Here's the drawing with two shaded views (mm, measured from the low corner). I have some questions. A direction names the side the tool comes from. Give positions to 0.01 mm unless a question says otherwise; leave off trailing zeros. Write each loop counter-clockwise with the first axis right and the second up, starting at its lowest first coordinate (ties: lowest second). Pieces come first, ordered by that corner, then holes.
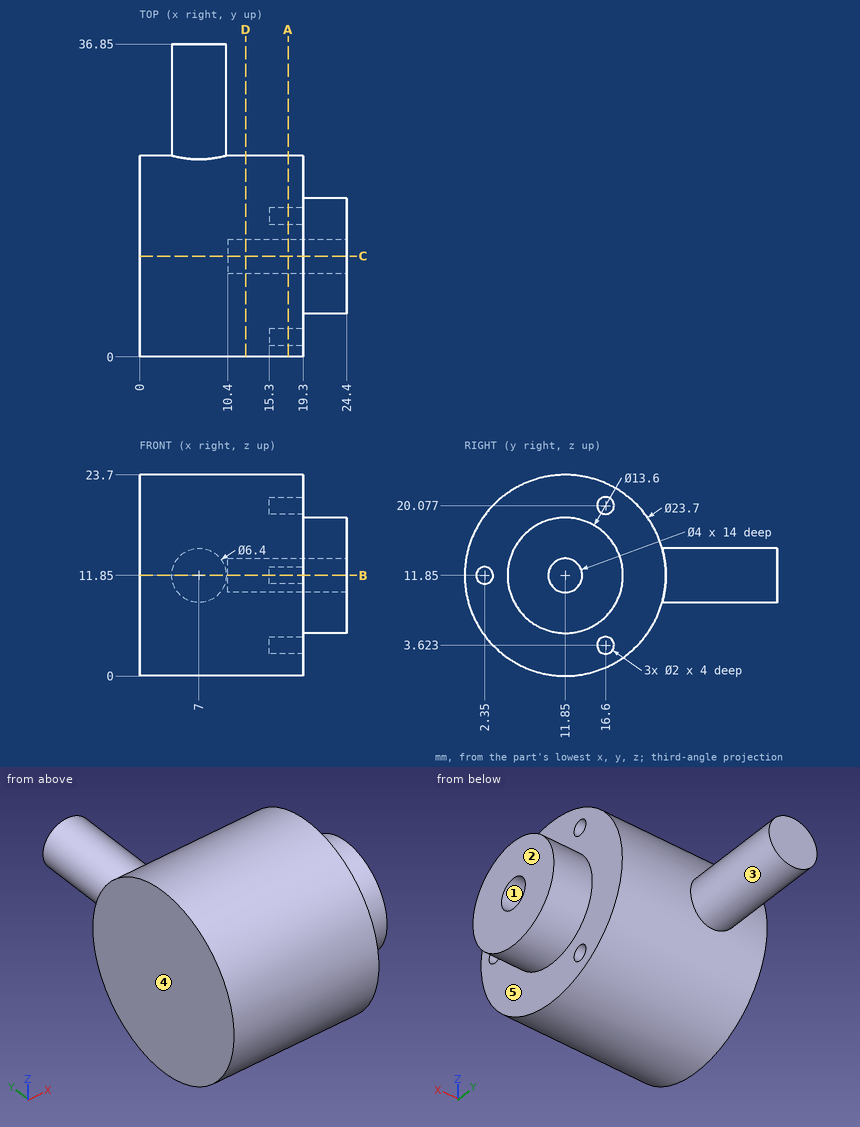
(1) Imagine slicing it at B-B, the plane z = 11.85. Write out the boundary of the cut face in (x, y), plus the area to 3 significant figures.
Returned:
outline: (0, 0) - (19.3, 0) - (19.3, 1.35) - (15.3, 1.35) - (15.3, 3.35) - (19.3, 3.35) - (19.3, 5.05) - (24.4, 5.05) - (24.4, 9.85) - (10.4, 9.85) - (10.4, 13.85) - (24.4, 13.85) - (24.4, 18.65) - (19.3, 18.65) - (19.3, 23.7) - (10.2, 23.7) - (10.2, 36.85) - (3.8, 36.85) - (3.8, 23.7) - (0, 23.7) - close
area: 547 mm2
(2) Imagine slicing it at C-C, the plane y = 11.85. Write out the boundary of the cut face in (x, z), plus the area to 3 significant figures.
Returned:
outline: (0, 0) - (19.3, 0) - (19.3, 5.05) - (24.4, 5.05) - (24.4, 9.85) - (10.4, 9.85) - (10.4, 13.85) - (24.4, 13.85) - (24.4, 18.65) - (19.3, 18.65) - (19.3, 23.7) - (0, 23.7) - close
area: 471 mm2
(3) If we mould it in two halves opening along Z, with no side actions, what happens to the marked faces 1, 2 and 3? For each: +Z half, -Z half, draft (parallel to the pull), parting line (faces both ways), or undercut.
Returned:
face 1: undercut
face 2: draft
face 3: parting line
(4) Will these pins go through, and if not, where does the flat tip stop? P1, Ø2.5, axis at y = 16.6, z = 20.08, coming from the +X side; P2, Ø1.5, axis at x = 12.5, z = 3.5, coming from the +Y side; P3, Ø1.6, axis at y = 16.6, z = 3.62, coming from the +X side; P4, Ø8, axis at x = 10, z = 15.5, coming from the -Y side.
Returned:
P1: stops at x = 19.3
P2: stops at y = 20.94
P3: stops at x = 15.3
P4: stops at y = 0
(5) Imagine slicing it at D-D, the plane x = 12.5. Write out the boundary of the cut face in (y, z), plus the area to 3 significant figures.
Returned:
outline: circle Ø23.7 at (11.85, 11.85); hole circle Ø4 at (11.85, 11.85)
area: 429 mm2
(6) Imagine slicing it at A-A, the plane x = 17.5. Write out the boundary of the cut face in (y, z), plus the area to 3 significant figures.
Returned:
outline: circle Ø23.7 at (11.85, 11.85); hole circle Ø2 at (2.35, 11.85); hole circle Ø4 at (11.85, 11.85); hole circle Ø2 at (16.6, 3.62); hole circle Ø2 at (16.6, 20.08)
area: 419 mm2
(7) If I drill on L1, parallel to X at y = 20.5, z = 17.5; L2, parallel to Y at x = 14.5, z = 7.75; L3, parallel to Y at x = 6, z = 5.25, over which ranges is the centre line in solid material (lowest first)?
Returned:
L1: x = 0 to 19.3
L2: y = 0.73 to 22.97
L3: y = 2.01 to 21.69
(8) For the marked faces 4 and 5, which set-ups out of +Z, -Z, +X, -X, +Y, -Y let a thin tool reach every point of the face, with its end or its side?
Returned:
face 4: +Z, -Z, -X, +Y, -Y
face 5: +X
